The model under review builds one solid part; all positions refer to its coordinate system, in mm. Face numbers are marked on the shaded views. A direction names the side the tool comes from. Give positions to 0.01 mm unless a question says otherwise; leave off trailing zeros. Order: outer loops, then holes, each group sorted by start corner. A loop starts at its lowest first (then second) coordinate and runs counter-clockwise, first axis right, second up. Notation, with made-up numbers: (24.25, 15.5) -> (52.25, 15.5) arc R13 cw to (52.25, 26.5) -> close; hole circle Ø6 at (2.25, 39). An arc over 180 degrees is marked (long way). Answer as a JSON object with one key per item and string values. Group by question number.
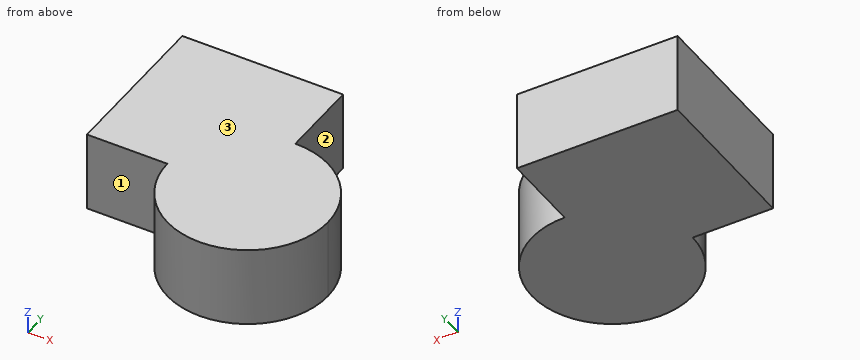
from build123d import *

# Parameters (mm, degrees)
F1_DEPTH = 25


with BuildPart() as f1:
    # F0 (on Top) → F1 (new body)
    with BuildSketch(Plane.XY):
        with BuildLine():
            ThreePointArc((39.129609, -3.07483), (31.807278, 14.60284), (14.129609, 21.92517))
            Line((14.129609, 21.92517), (14.129609, -3.07483))
            Line((14.129609, -3.07483), (-10.870391, -3.07483))
            ThreePointArc((-10.870391, -3.07483), (14.129609, -28.07483), (39.129609, -3.07483))
        make_face()
        with BuildLine():
            Line((14.129609, -3.07483), (14.129609, 21.92517))
            ThreePointArc((14.129609, 21.92517), (-3.548061, 14.60284), (-10.870391, -3.07483))
            Line((-10.870391, -3.07483), (14.129609, -3.07483))
        make_face()
        with BuildLine():
            Line((14.129609, 46.92517), (-35.870391, 46.92517))
            Line((-35.870391, 46.92517), (-35.870391, -3.07483))
            Line((-35.870391, -3.07483), (-10.870391, -3.07483))
            ThreePointArc((-10.870391, -3.07483), (-3.548061, 14.60284), (14.129609, 21.92517))
            Line((14.129609, 21.92517), (14.129609, 46.92517))
        make_face()
    extrude(amount=F1_DEPTH)


solid = f1.part
1. Take a section at B-B on x = -30.5. Give the boundary of the cut face in (y, z), plus the area to 3 significant figures.
2. Take a section at A-A on z = 10.5. Give the boundary of the cut face in (x, y), plus the area to 3 significant figures.
3. Machinability: for the marked faces 1, 2 and 3, which of the approach directions +Z, -Z, +X, -X, +Y, -Y give a long, thin tool a straight path to every point of the face, cutting with its end or side? Answer none if there is none.
4. Take a section at C-C on y = 34.5. Give the boundary of the cut face in (x, z), plus the area to 3 significant figures.
5. For probe 1 along X at (y, z) = (29, 9.75); probe 2 along Y at (x, z) = (-23, 9.5); probe 3 along Y at (x, z) = (19.5, 1.75), list the stretches that pass through material, from the lowest coordinate up. Write a range as [from, to].
6. For pin 1 (1 mm diameter, centred on y = -8, z = 22.5, fed in from +X); pin 2 (12.5 mm diameter, centred on x = -21, z = 15, fed in from -Y); pin 3 (2 mm diameter, centred on y = 26, z = 10, fed in from +X), all flat-tipped, find the tip position at first contact; note any pin that passes through.
Checks:
{
 "1": {"outline": "(-3.07, 0) -> (46.93, 0) -> (46.93, 25) -> (-3.07, 25) -> close", "area": "1,250 mm2"},
 "2": {"outline": "(-35.87, -3.07) -> (-10.87, -3.07) arc R25 ccw (long way) to (14.13, 21.93) -> (14.13, 46.93) -> (-35.87, 46.93) -> close", "area": "3,970 mm2"},
 "3": {"face 1": "+Z, -Z, -X, -Y", "face 2": "+Z, -Z, +X, +Y", "face 3": "+Z, +X, -X, +Y, -Y"},
 "4": {"outline": "(-35.87, 0) -> (14.13, 0) -> (14.13, 25) -> (-35.87, 25) -> close", "area": "1,250 mm2"},
 "5": {"probe 1": "x = [-35.87, 14.13]", "probe 2": "y = [-3.07, 46.93]", "probe 3": "y = [-27.49, 21.34]"},
 "6": {"pin 1": "stops at x = 38.73", "pin 2": "stops at y = -3.07", "pin 3": "stops at x = 14.13"}
}
